Autodesk Inventor part; units mm, degrees
ref_plane "Work Plane1" through (0, 0, -127) normal (0, 0, 1) x (1, 0, 0)
ref_plane "YZ Plane" through (0, 0, 0) normal (1, 0, 0) x (0, 1, 0)
ref_plane "XZ Plane" through (0, 0, 0) normal (0, 1, 0) x (-1, 0, 0)
sketch "Sketch1" plane through (0, 0, 0) normal (0, 1, 0) x (-1, 0, 0)
  line L0 (0, 0) -> (-63.5, 0)
  line L1 (-63.5, 0) -> (-63.5, -254)
  line L2 (-63.5, -254) -> (0, -254)
  line L3 (0, -254) -> (0, 0)
  dimension "d0" = 63.5
  dimension "d1" = 254
extrude "Extrusion1" add sketch "Sketch1" along normal blind 3.81
sketch "Sketch2" plane through (0, 3.81, 0) normal (0, 1, 0) x (1, 0, 0)
  line L0 (0, 254) -> (0, 0)
  line L1 (0, 0) -> (63.5, 0)
  line L2 (63.5, 0) -> (63.5, 254)
  line L3 (63.5, 254) -> (0, 254)
  line L4 (3.175, 3.175) -> (3.175, 250.825)
  line L5 (3.175, 250.825) -> (60.325, 250.825)
  line L6 (60.325, 250.825) -> (60.325, 3.175)
  line L7 (60.325, 3.175) -> (3.175, 3.175)
  line L8 (3.175, 3.175) -> (60.325, 3.175)
  line L9 (60.325, 3.175) -> (60.325, 52.705)
  line L10 (60.325, 52.705) -> (3.175, 52.705)
  line L11 (3.175, 52.705) -> (3.175, 3.175)
  line L12 (3.175, 3.175) -> (3.175, 6.731)
  line L13 (3.175, 6.731) -> (29.5398, 27.94)
  line L14 (60.325, 52.705) -> (60.325, 49.149)
  line L15 (60.325, 49.149) -> (33.9602, 27.94)
  line L16 (3.175, 52.705) -> (3.175, 49.149)
  line L17 (3.175, 49.149) -> (29.5398, 27.94)
  line L18 (60.325, 3.175) -> (60.325, 6.731)
  line L19 (60.325, 6.731) -> (33.9602, 27.94)
  line L20 (31.75, 26.162) -> (3.175, 3.175)
  line L21 (31.75, 29.718) -> (3.175, 52.705)
  line L22 (31.75, 26.162) -> (60.325, 3.175)
  line L23 (31.75, 29.718) -> (60.325, 52.705)
  point P0 (60.325, 3.175)
  dimension "d4" = 3.175
  dimension "d5" = 49.53
  dimension "d6" = 3.556
  dimension "d7" = 3.556
  dimension "d8" = 3.556
  dimension "d9" = 3.556
extrude "Extrusion2" cut sketch "Sketch2" against normal blind 6.35 contours L20 L22 L7 | L4 L17 L13 | L19 L15 L6 | L10 L23 L21
pattern_linear "Rectangular Pattern1" count 5 spacing 49.53 along (0, 0, -1) of "Extrusion2"
sketch "Sketch4" plane through (0, 3.81, 0) normal (0, 1, 0) x (1, 0, 0)
  line L0 (33.9602, 27.94) -> (60.325, 6.731)
  line L1 (3.175, 6.731) -> (29.5398, 27.94)
  line L2 (60.325, 6.731) -> (3.175, 6.731)
  line L3 (3.175, 3.175) -> (60.325, 3.175)
  line L4 (3.175, 6.731) -> (3.175, 3.175)
  line L5 (3.175, 3.175) -> (60.325, 3.175)
  line L6 (60.325, 6.731) -> (60.325, 49.149)
  line L7 (60.325, 3.175) -> (60.325, 6.731)
  point P0 (0, 0)
extrude "Extrusion3" add sketch "Sketch4" against normal blind 3.81
sketch "Sketch3" plane through (63.5, 0, 0) normal (1, 0, 0) x (0, 0, -1)
  line L0 (3.175, 3.81) -> (3.175, 0)
  point P0 (0, 0)
  point P1 (3.175, 1.905)
  dimension "d15" = 0
hole "Hole1" at (63.5, 1.905, -3.175) direction (-1, 0, 0) diameter 2.4384 end through all
ref_plane "Work Plane1" through (0, 0, -127) normal (0, 0, 1) x (1, 0, 0)
mirror "Mirror1" about plane through (0, 0, -127) normal (0, 0, 1) of "Extrusion3", "Hole1"
fillet "Fillet1" radius 1.27 4 edges at (31.75, 3.81, 0) (31.75, 0, 0) (31.75, 3.81, -254) (31.75, 0, -254)
sketch "Sketch5" plane through (0, 3.81, 0) normal (0, 1, 0) x (1, 0, 0)
  line L0 (3.175, 52.705) -> (31.75, 29.718)
  line L1 (3.175, 52.705) -> (60.325, 52.705)
  line L2 (60.325, 52.705) -> (60.325, 0)
  line L3 (60.325, 0) -> (3.175, 0)
  line L4 (3.175, 0) -> (3.175, 52.705)
  line L5 (60.325, 49.149) -> (60.325, 6.731)
  line L6 (0, 0) -> (63.5, 0)
extrude "Extrusion4" cut sketch "Sketch5" against normal blind 3.81
properties part number "ferris_wheel_main_strut"
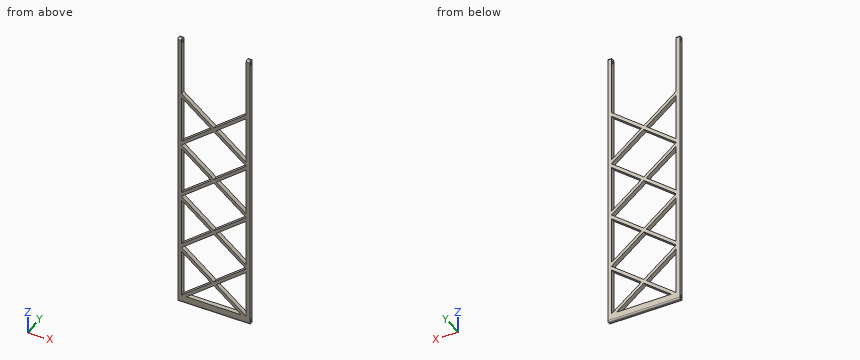
Geometry: final body of the model. Coordinates: model frame, mm. Round coordinates to 2 decimals unless told otherwise and drop trailing zeros. Loops run counter-clockwise (first coordinate to the right, second up) from the corner with the lowest first, then second, coordinate; pieces in that order, holes last. Notation, with made-up numbers: M -2,53 L 18,53 A21 ccw 18,70 Z; hole C -12,-33 d3. An arc over 180 degrees is marked long. Put each result on its own line as item: value. Start each with the question number.
(1) Section query A-A (z = -234). Return loops of the section in (x, y) (3 decimals).
(2) Section query B-B (x = 5.5). State how many separate pieces and enclosed holes the cut face has, then the cut area to 3 significant figures.
(3) Material intervals for line 1 along X through (y, z) = (3.2, -160) (3 decimals); line 2 along X through (y, z) = (3.65, -136) (3 decimals); line 3 along X through (y, z) = (1.85, -31) (3 decimals), sorted ascending. Write a range as [from, to].
Findings below:
1. outline: M 0,0 L 3.175,0 L 3.175,3.81 L 0,3.81 Z; M 19.67,0 L 24.09,0 L 24.09,3.81 L 19.67,3.81 Z; M 39.41,0 L 43.83,0 L 43.83,3.81 L 39.41,3.81 Z; M 60.325,0 L 63.5,0 L 63.5,3.81 L 60.325,3.81 Z
2. separate pieces: 8
2. enclosed holes: 1
2. area: 122 mm2
3. line 1: x = [0, 3.175], [8.991, 13.412], [50.088, 54.509], [60.325, 63.5]
3. line 2: x = [0, 3.175], [18.352, 22.772], [40.728, 45.148], [60.325, 63.5]
3. line 3: x = [0, 3.175], [60.325, 63.5]
